Autodesk Inventor part; units mm, degrees
ref_plane "YZ Plane" through (0, 0, 0) normal (1, 0, 0) x (0, 1, 0)
ref_plane "XZ Plane" through (0, 0, 0) normal (0, 1, 0) x (-1, 0, 0)
ref_plane "XY Plane" through (0, 0, 0) normal (0, 0, 1) x (1, 0, 0)
sketch "Эскиз1" plane through (0, 0, 0) normal (0, 0, 1) x (1, 0, 0)
  line L0 (0, 0) -> (390, 0)
  line L1 (390, 0) -> (390, 227)
  line L2 (390, 227) -> (0, 227)
  line L3 (0, 227) -> (0, 0)
  line L4 (4, 223) -> (386, 223)
  line L5 (386, 223) -> (386, 8)
  line L6 (386, 8) -> (4, 8)
  line L7 (4, 8) -> (4, 223)
  line L8 (51.2, 0) -> (338.8, 0)
  line L9 (338.8, 0) -> (338.8, -11)
  line L10 (338.8, -11) -> (51.2, -11)
  line L11 (51.2, -11) -> (51.2, 0)
  line L12 (195, 8) -> (195, 37.2602)
  point P0 (195, 223)
  point P1 (195, 227)
  point P2 (195, -11)
  dimension "d0" = 390
  dimension "d1" = 227
  dimension "d2" = 382
  dimension "d3" = 215
  dimension "d4" = 4
  dimension "d5" = 8
  dimension "d6" = 4
  dimension "d7" = 238
  dimension "d9" = 287.6
extrude "Выдавливание1" add sketch "Эскиз1" along normal blind 3.5
sketch "Эскиз2" plane through (0, 0, 3.5) normal (0, 0, 1) x (1, 0, 0)
  line L0 (0, 0) -> (51.2, 0)
  line L1 (51.2, 0) -> (51.2, -11)
  line L2 (51.2, -11) -> (338.8, -11)
  line L3 (338.8, -11) -> (338.8, 0)
  line L4 (338.8, 0) -> (390, 0)
  line L5 (390, 0) -> (390, 227)
  line L6 (390, 227) -> (0, 227)
  line L7 (0, 227) -> (0, 0)
  line L8 (386, 223) -> (386, 8)
  line L9 (386, 8) -> (4, 8)
  line L10 (4, 8) -> (4, 223)
  line L11 (4, 223) -> (386, 223)
extrude "Выдавливание2" add sketch "Эскиз2" against normal blind 3.4 contours L8 L9 L10 L11
sketch "Эскиз3" plane through (0, 0, 0) normal (0, 0, -1) x (-1, 0, 0)
  line L0 (0, 0) -> (-51.2, 0)
  line L1 (0, 227) -> (0, 0)
  line L2 (-390, 227) -> (0, 227)
  line L3 (-390, 0) -> (-390, 227)
  line L4 (-338.8, 0) -> (-390, 0)
  line L5 (-338.8, -11) -> (-338.8, 0)
  line L6 (-51.2, -11) -> (-338.8, -11)
  line L7 (-51.2, 0) -> (-51.2, -11)
  line L8 (-386, 223) -> (-386, 8)
  line L9 (-4, 223) -> (-386, 223)
  line L10 (-4, 8) -> (-4, 223)
  line L11 (-386, 8) -> (-4, 8)
  line L12 (-195, -11) -> (-195, 1.1845)
  line L13 (-255.24, 5) -> (-230.3, 5)
  line L14 (-230.3, 5) -> (-230.3, 3)
  line L15 (-230.3, 3) -> (-255.24, 3)
  line L16 (-255.24, 3) -> (-255.24, 5)
  line L17 (-338.98, 5) -> (-314.04, 5)
  line L18 (-314.04, 5) -> (-314.04, 3)
  line L19 (-314.04, 3) -> (-338.98, 3)
  line L20 (-338.98, 3) -> (-338.98, 5)
  line L21 (-134.76, 5) -> (-159.7, 5)
  line L22 (-159.7, 5) -> (-159.7, 3)
  line L23 (-159.7, 3) -> (-134.76, 3)
  line L24 (-134.76, 3) -> (-134.76, 5)
  line L25 (-51.02, 5) -> (-75.96, 5)
  line L26 (-75.96, 5) -> (-75.96, 3)
  line L27 (-75.96, 3) -> (-51.02, 3)
  line L28 (-51.02, 3) -> (-51.02, 5)
  point P0 (-314.04, 4)
  point P1 (-255.24, 4)
  point P2 (-75.96, 4)
  point P3 (-134.76, 4)
  dimension "d14" = 24.94
  dimension "d15" = 35.3
  dimension "d16" = 3
  dimension "d17" = 2
  dimension "d18" = 2
  dimension "d19" = 24.94
  dimension "d20" = 58.8
extrude "Выдавливание3" cut sketch "Эскиз3" against normal blind 1 contours L13 L14 L15 L16 | L17 L18 L19 L20 | L24 L23 L22 L21 | L28 L27 L26 L25
sketch "Эскиз5" plane through (0, 0, 3.5) normal (0, 0, 1) x (1, 0, 0)
  line L0 (0, 0) -> (51.2, 0)
  line L1 (51.2, 0) -> (51.2, -11)
  line L2 (51.2, -11) -> (338.8, -11)
  line L3 (338.8, -11) -> (338.8, 0)
  line L4 (338.8, 0) -> (390, 0)
  line L5 (390, 0) -> (390, 227)
  line L6 (390, 227) -> (0, 227)
  line L7 (0, 227) -> (0, 0)
  line L8 (230.5, -11) -> (265.5, -11)
  line L9 (265.5, -11) -> (265.5, 9)
  line L10 (265.5, 9) -> (230.5, 9)
  line L11 (230.5, 9) -> (230.5, -11)
  dimension "d23" = 124.5
  dimension "d24" = 20
  dimension "d25" = 35
extrude "Выдавливание4" cut sketch "Эскиз5" against normal blind 1 contours L11 L10 L9 L2
equation "\"d19\" = d14"
properties part number "NV173FHM-N4G V8.0"
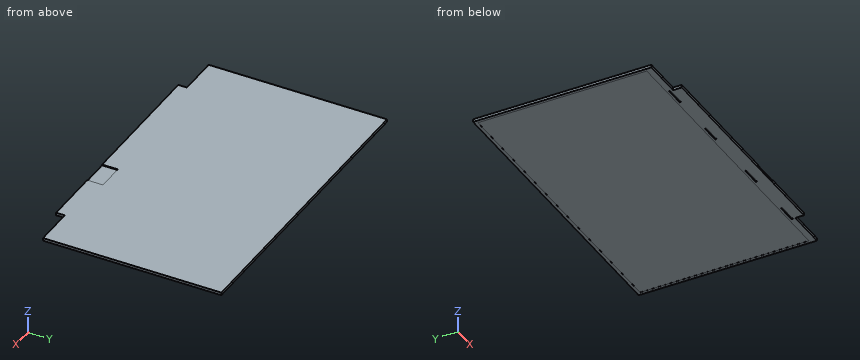
Read the model definition and answer for the solid it produces. Units are mm, in the model's axes. Round coordinates to 2 decimals unless told otherwise and drop trailing zeros. Order: outer loops, then holes, each group sorted by start corner. A loop starts at its lowest first (then second) coordinate and runs counter-clockwise, first axis right, second up.
1) The part is cut by section B-B on y = 161. Write down the section's boundary in (x, z), plus the area to 3 significant figures.
2) The part is cut by section C-C on x = 61. Write down the section's boundary in (y, z), plus the area to 4 significant figures.
3) Flat-ended cylindrical pins translate along their axes: pin 1 (1 mm diameter, centred on x = 240.5, y = 4, fed in from -Z); pin 2 (6 mm diameter, centred on x = 344.5, y = 16.5, fed in from -Z); pin 3 (22 mm diameter, centred on x = 248, y = -3, fed in from +Z). Find the tip coordinate at first contact, or state that the pin passes through.
4) The part is cut by section A-A on x = 351.5. Write down the section's boundary in (y, z).
5) Straight lines are drawn through the part: L1, parallel to Y at x = 31, z = 1.6; L2, parallel to Z at x = 143, y = 129.5. For each, find the intervals that lie inside material, in ascending order.
Resolved:
1. outline: (0, 0) - (4, 0) - (4, 0.1) - (386, 0.1) - (386, 0) - (390, 0) - (390, 3.5) - (0, 3.5) - close
1. area: 1,330 mm2
2. outline: (-11, 0) - (3, 0) - (3, 1) - (5, 1) - (5, 0) - (8, 0) - (8, 0.1) - (223, 0.1) - (223, 0) - (227, 0) - (227, 3.5) - (-11, 3.5) - close
2. area: 809.5 mm2
3. pin 1: stops at z = 1
3. pin 2: stops at z = 0.1
3. pin 3: stops at z = 2.5
4. outline: (0, 0) - (8, 0) - (8, 0.1) - (223, 0.1) - (223, 0) - (227, 0) - (227, 3.5) - (0, 3.5) - close
5. L1: y = 0 to 227
5. L2: z = 0.1 to 3.5
